Autodesk Inventor part; units mm, degrees
ref_plane "YZ Plane" through (0, 0, 0) normal (1, 0, 0) x (0, 1, 0)
ref_plane "XZ Plane" through (0, 0, 0) normal (0, 1, 0) x (-1, 0, 0)
ref_plane "XY Plane" through (0, 0, 0) normal (0, 0, 1) x (1, 0, 0)
sketch "Sketch3" plane through (0, 0, 0) normal (0, 1, 0) x (-1, 0, 0)
  line L0 (0, -300) -> (0, 0)
  line L1 (68.5, 0) -> (68.5, -75)
  line L2 (68.5, -75) -> (98.5, -75)
  line L3 (68.5, -300) -> (68.5, -225)
  line L4 (68.5, -225) -> (98.5, -225)
  line L5 (0, 0) -> (68.5, 0)
  line L6 (68.5, 0) -> (68.5, -75)
  line L7 (68.5, -75) -> (98.5, -75)
  line L8 (98.5, -75) -> (98.5, -225)
  line L9 (0, -300) -> (68.5, -300)
  circle A0 centre (88.5, -105) radius 6.5
  circle A1 centre (88.5, -135) radius 6.5
  circle A2 centre (88.5, -165) radius 6.5
  circle A3 centre (88.5, -195) radius 6.5
  dimension "d44" = 30
  dimension "d48" = 13
  dimension "d49" = 30
  dimension "d50" = 10
  dimension "d56" = 30
  dimension "d70" = 150
  dimension "d71" = 75
  dimension "d72" = 75
  dimension "d73" = 68.5
  dimension "d74" = 68.5
  dimension "d75" = 68.5
  dimension "d76" = 30
  dimension "d77" = 150
  dimension "d78" = 90
  dimension "d79" = 90
extrude "Extrusion1" add sketch "Sketch3" along normal blind 50.8
sketch "Sketch6" plane through (0, 50.8, 0) normal (0, 1, 0) x (1, 0, 0)
  line L0 (-98.5, 225) -> (-98.5, 75)
  line L1 (-98.5, 102.5) -> (-93.5, 102.5)
  line L2 (-93.5, 102.5) -> (-93.5, 107.5)
  line L3 (-93.5, 107.5) -> (-98.5, 107.5)
  line L4 (-98.5, 107.5) -> (-98.5, 102.5)
  circle A0 centre (-88.5, 105) radius 6.5
  line L5 (-93.5, 132.5) -> (-93.5, 137.5)
  line L6 (-93.5, 137.5) -> (-98.5, 137.5)
  line L7 (-98.5, 137.5) -> (-98.5, 132.5)
  line L8 (-98.5, 132.5) -> (-93.5, 132.5)
  line L9 (-93.5, 162.5) -> (-93.5, 167.5)
  line L10 (-93.5, 167.5) -> (-98.5, 167.5)
  line L11 (-98.5, 167.5) -> (-98.5, 162.5)
  line L12 (-98.5, 162.5) -> (-93.5, 162.5)
  line L13 (-93.5, 192.5) -> (-93.5, 197.5)
  line L14 (-93.5, 197.5) -> (-98.5, 197.5)
  line L15 (-98.5, 197.5) -> (-98.5, 192.5)
  line L16 (-98.5, 192.5) -> (-93.5, 192.5)
  point P0 (0, 0)
  dimension "d58" = 5
  dimension "d59" = 5
  dimension "d60" = 2.5
  dimension "d66" = 30
extrude "Extrusion3" cut sketch "Sketch6" against normal blind 50.8 contours L14 L13 L16 L0 | L3 A0 L1 L0 | L6 L5 L8 L0 | L10 L9 L12 L0 | L3 L2 L1 A0 picked at (-94, 105)
properties part number "PiezaInferior"
The listing builds one solid part. Answer for the finished solid, in the listing's coordinates (mm). A direction names the side the tool comes from. Give positions to 0.01 mm unless a question says otherwise; leave off trailing zeros. Order: outer loops, then holes, each group sorted by start corner. A loop starts at its lowest first (then second) coordinate and runs counter-clockwise, first axis right, second up. Notation, with made-up numbers: (-8, -2) -> (23, -2) arc R21 cw to (23, 20) -> close; hole circle Ø1 at (48, -15). An arc over 180 degrees is marked (long way). Answer as a JSON object with one key per item and string values. Group by question number.
Item 1: Flat-ended cylindrical pins translate along their axes: pin 1 (3 mm diameter, centred on x = -96, y = 20.5, fed in from -Z); pin 2 (10.5 mm diameter, centred on x = -88.5, z = -105, fed in from +Y); pin 3 (2 mm diameter, centred on x = -96, y = 31.5, fed in from +Z); pin 4 (15 mm diameter, centred on y = 36.5, z = -279.5, fed in from -X). Find the tip coordinate at first contact, or state that the pin passes through.
Item 2: Determine the mould class of faces 4 (the cylindrical face through (-82, 25, -135)), 5 (the flat face through (-98.5, 25, -120)), 6 (the flat face through (-83, 25, -75)) for opening direction Z: pulls with the +Z half, pulls with the -Z half, needs draft (parallel to the pull), parting line crosses it, or undercut.
Item 3: The part is cut by section C-C on z = -257. Write down the section's boundary in (x, y).
Item 4: A tool of negligible diameter and unlimited length cuts with its end or side. For faces 1 (the flat face through (-68.5, 25, -37)), 2 (the flat face through (-83, 25, -225)), 3 (the flat face through (-98.5, 25, -89)), from which of +Z, -Z, +X, -X, +Y, -Y can it reach the whole face along a straight path? Write none if from no direction.
Item 5: The part is cut by section A-A on x = -88.5. Write down the section's boundary in (y, z).
Item 6: Consider L1, parallel to Z at x = -88, y = 22; L2, parallel to X at y = 22.5, z = -13; L3, parallel to Z at x = -90.5, y = 19. Determine where each line is inside the solid, lowest interval first. Write a range as from..to.
Item 7: The part is cut by section B-B on y = 18.5. Write down the section's boundary in (x, z), and give its area (3 significant figures).
Result set:
{
 "1": {"pin 1": "z = -225", "pin 2": "through", "pin 3": "z = -75", "pin 4": "x = -68.5"},
 "2": {"face 4": "undercut", "face 5": "needs draft", "face 6": "pulls with the +Z half"},
 "3": {"outline": "(-68.5, 0) -> (0, 0) -> (0, 50.8) -> (-68.5, 50.8) -> close"},
 "4": {"face 1": "+Z, -X, +Y, -Y", "face 2": "-Z, -X, +Y, -Y", "face 3": "+Z, -Z, -X, +Y, -Y"},
 "5": {"outline": "(0, -225) -> (50.8, -225) -> (50.8, -201.5) -> (0, -201.5) -> close; (0, -188.5) -> (50.8, -188.5) -> (50.8, -171.5) -> (0, -171.5) -> close; (0, -158.5) -> (50.8, -158.5) -> (50.8, -141.5) -> (0, -141.5) -> close; (0, -128.5) -> (50.8, -128.5) -> (50.8, -111.5) -> (0, -111.5) -> close; (0, -98.5) -> (50.8, -98.5) -> (50.8, -75) -> (0, -75) -> close"},
 "6": {"L1": "-225..-201.48, -188.52..-171.48, -158.52..-141.48, -128.52..-111.48, -98.52..-75", "L2": "-68.5..0", "L3": "-225..-201.18, -188.82..-171.18, -158.82..-141.18, -128.82..-111.18, -98.82..-75"},
 "7": {"outline": "(-98.5, -225) -> (-68.5, -225) -> (-68.5, -300) -> (0, -300) -> (0, 0) -> (-68.5, 0) -> (-68.5, -75) -> (-98.5, -75) -> (-98.5, -102.5) -> (-94.5, -102.5) arc R6.5 cw (long way) to (-94.5, -107.5) -> (-98.5, -107.5) -> (-98.5, -132.5) -> (-94.5, -132.5) arc R6.5 cw (long way) to (-94.5, -137.5) -> (-98.5, -137.5) -> (-98.5, -162.5) -> (-94.5, -162.5) arc R6.5 cw (long way) to (-94.5, -167.5) -> (-98.5, -167.5) -> (-98.5, -192.5) -> (-94.5, -192.5) arc R6.5 cw (long way) to (-94.5, -197.5) -> (-98.5, -197.5) -> close", "area": "24,400 mm²"}
}
